Can you work these out from the model? Positions are in its coordinate system, mm. Face numbers are marked on the shaded views. A direction names the side the tool comes from. Coordinates: 2 decimals unless noted, no trailing zeros. Loops run counter-clockwise (first coordinate to the right, second up) from the corner with the lowest first, then second, coordinate; pieces in that order, holes last.
```python
from build123d import *

# Parameters (mm, degrees)
SKETCH1_W                 = 140
SKETCH1_H                 = 50
BOSS_EXTRUDE1_DEPTH       = 10
BOSS_EXTRUDE2_START       = -12.5
BOSS_EXTRUDE2_DEPTH       = 35
CUT_EXTRUDE1_DEPTH        = 50
BOSS_EXTRUDE8_DEPTH       = 5
BOSS_EXTRUDE9_START       = -18.443977
BOSS_EXTRUDE9_OUTLINE_R   = 25
BOSS_EXTRUDE9_OUTLINE_R_2 = 12.5
BOSS_EXTRUDE9_DEPTH       = 30
FILLET1_R                 = 18
CUT_EXTRUDE2_START        = -30
CUT_EXTRUDE2_DEPTH        = 30


# Read off the part's stored shape, not the designer's step: Boss-Extrude2, Boss-Extrude9
with BuildPart() as part:
    # Sketch1 → Boss-Extrude1 (new body)
    with BuildSketch(Plane(origin=(0, 0, 0), x_dir=(1, 0, 0), z_dir=(0, 1, 0))):
        with Locations((17.140882, 3.443977)):
            Rectangle(SKETCH1_W, SKETCH1_H)
    extrude(amount=BOSS_EXTRUDE1_DEPTH)

    # Boss-Extrude2 outline → Boss-Extrude2 (add)
    with BuildSketch(Plane(origin=(0, 0, 0), x_dir=(1, 0, 0), z_dir=(0, 1, 0)).offset(BOSS_EXTRUDE2_START)):
        with BuildLine():
            Line((-51.363996, 28.275018), (-52.859118, 28.275018))
            Line((-52.859118, 28.275018), (-74.973336, 28.275018))
            ThreePointArc((-74.973336, 28.275018), (-102.814942, 4.885934), (-77.856685, -21.558151))
            Line((-77.856685, -21.558151), (-52.858882, -21.680248))
            ThreePointArc((-52.858882, -21.680248), (-27.870068, 2.571974), (-51.363996, 28.275018))
        make_face()
        with BuildLine():
            Line((-52.859118, 13.319754), (-52.858882, 13.319753))
            ThreePointArc((-52.858882, 13.319753), (-42.85888, 3.319752), (-52.858882, -6.68025))
            Line((-52.858882, -6.68025), (-52.859118, -6.680248))
            Line((-52.859118, -6.680248), (-77.856685, -6.558153))
            ThreePointArc((-77.856685, -6.558153), (-87.856686, 3.441849), (-77.856685, 13.44185))
            Line((-77.856685, 13.44185), (-52.859118, 13.319754))
        make_face(mode=Mode.SUBTRACT)
    extrude(amount=BOSS_EXTRUDE2_DEPTH)

    # Sketch2 → Cut-Extrude1 (cut)
    with BuildSketch(Plane(origin=(0, 10, 0), x_dir=(1, 0, 0), z_dir=(0, 1, 0))):
        with BuildLine():
            Line((-52.859118, 13.319753), (-52.859118, -6.68025))
            ThreePointArc((-52.859118, -6.68025), (-42.859116, 3.319752), (-52.859118, 13.319753))
        make_face()
    extrude(amount=-CUT_EXTRUDE1_DEPTH, mode=Mode.SUBTRACT)

    # 3DSketch2 → Boss-Extrude8 (add, symmetric)
    with BuildSketch(Plane(origin=(87.140882, 10, -3.443977), x_dir=(-0.9975892937431798, 0.0693945315495666, 0), z_dir=(0, 0, -1))):
        Polygon((0, 0), (114.733361, -7.981108), (115.288545, 0), (50.434648, 4.511381), (53.730889, 51.896873), (3.851424, 55.366599), align=None)
    extrude(amount=BOSS_EXTRUDE8_DEPTH, both=True)

    # Boss-Extrude9 outline → Boss-Extrude9 (add)
    with BuildSketch(Plane.XY.offset(BOSS_EXTRUDE9_START)):
        with Locations((62.140882, 65.500395)):
            Circle(BOSS_EXTRUDE9_OUTLINE_R)
        with Locations((62.140882, 65.500395)):
            Circle(BOSS_EXTRUDE9_OUTLINE_R_2, mode=Mode.SUBTRACT)
    extrude(amount=BOSS_EXTRUDE9_DEPTH)

    # Fillet1
    fillet1_edges = [part.edges().sort_by_distance(p)[0] for p in [
        (37.140882, 18.000395, -3.443977),
    ]]
    fillet(fillet1_edges, radius=FILLET1_R)

    # Sketch3 → Cut-Extrude2 (cut)
    with BuildSketch(Plane.XY.offset(1.556023).offset(CUT_EXTRUDE2_START)):
        with BuildLine():
            Line((74.640882, 65.500395), (49.640882, 65.500395))
            ThreePointArc((49.640882, 65.500395), (62.140882, 53.000395), (74.640882, 65.500395))
        make_face()
    extrude(amount=CUT_EXTRUDE2_DEPTH, mode=Mode.SUBTRACT)


solid = part.part
```
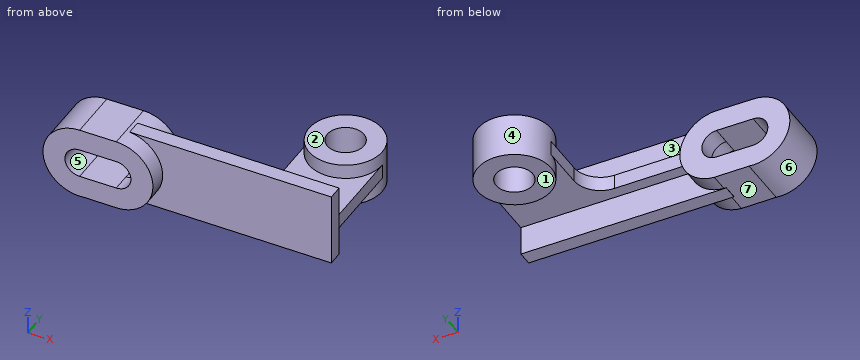
Item 1: We'd pull the mould along Z, two halves only. Please class the marked faces 4, 5, 6 and 7: +Z half, -Z half, draft (parallel to the pull), parting line (faces both ways), or undercut.
Results are:
face 4: draft
face 5: undercut
face 6: parting line
face 7: -Z half
Item 2: Suppose I cut it at C-C, the plane x = 60. Please give me the cut outline in (y, z).
Results are:
outline: (0, -28.44) - (10, -28.44) - (10, -8.44) - (40.59, -8.44) - (40.59, -18.44) - (53.19, -18.44) - (53.19, 11.56) - (40.59, 11.56) - (40.59, 1.56) - (10, 1.56) - (10, 21.56) - (0, 21.56) - close; (77.82, -18.44) - (90.41, -18.44) - (90.41, 11.56) - (77.82, 11.56) - close
Item 3: On a 3-axis mill with a long thin cutter (end or side, diameter ignored), from which of +Z, -Z, +X, -X, +Y, -Y can I reach the whole of each face in a straight line? I mean the marked faces 1, 2 and 3. Say none if no direction works.
Results are:
face 1: -Z, +X, -X, +Y
face 2: +Z, +X, -X, +Y
face 3: +Z, +X
Item 4: Suppose I cut it at D-D, the plane x = 12. Please give me the cut outline in (y, z), plus the area to 3 significant figures.
Results are:
outline: (0, -28.44) - (10, -28.44) - (10, -8.44) - (18, -8.44) - (18, 1.56) - (10, 1.56) - (10, 21.56) - (0, 21.56) - close
area: 580 mm2
Item 5: I need wall thicknesses on line 1 along X through (y, z) = (6, -3.5); line 2 along Y through (x, z) = (-46.5, 12.5); line 3 along Y through (x, z) = (37, 4). Which ranges of each line are inside material? Lowest first, please.
Results are:
line 1: x = -102.86 to -87.86, -42.86 to 87.14
line 2: y = -12.5 to 22.5
line 3: y = 0 to 10
Item 6: Suppose I cut it at B-B, the plane z = 3.5. Count the separate pieces of the cut face and the enclosed holes in it, plus the area to 3 significant figures.
Results are:
separate pieces: 3
enclosed holes: 1
area: 3,810 mm2
Item 7: I'm going to push flat-ended pins straight in: P1, Ø25, axis at x = 66.5, y = 69.5, coming from the -Z side; P2, Ø4, axis at x = -38, z = -22, coming from the +Y side; P3, Ø1.5, axis at x = 33, z = 9.5, coming from the -Y side. Where does each tip first touch, or does it pass through?
Results are:
P1: stops at z = -18.44
P2: stops at y = 22.5
P3: stops at y = 0
